Verification items for the finished model (mm, model axes). A direction names the side the tool comes from. Round coordinates to 2 decimals unless told otherwise and drop trailing zeros. Loops run counter-clockwise (first coordinate to the right, second up) from the corner with the lowest first, then second, coordinate; pieces in that order, holes last. Notation, with made-up numbers: M -11,-17.5 L -7,-17.5 A25 ccw -7,19.5 Z; hole C 43.5,-4.5 d6. An arc over 180 degrees is marked long. Answer as CSV lines item,"result".
```python
from build123d import *

# Parameters (mm, degrees)
TUBO_CUADRADO_40_X_40_X_4_1_DEPTH = 600
CROQUIS3_R                        = 4
CORTAR_EXTRUIR1_DEPTH             = 25


with BuildPart() as part:
    # Sketch1 → Tubo cuadrado 40 X 40 X 4(1) (new body)
    with BuildSketch(Plane(origin=(-300, 0, 0), x_dir=(0, 0, -1), z_dir=(1, 0, 0))):
        with BuildLine():
            Line((-12, -20), (12, -20))
            ThreePointArc((12, -20), (17.656854249, -17.656854249), (20, -12))
            Line((20, -12), (20, 12))
            ThreePointArc((20, 12), (17.656854249, 17.656854249), (12, 20))
            Line((12, 20), (-12, 20))
            ThreePointArc((-12, 20), (-17.656854249, 17.656854249), (-20, 12))
            Line((-20, 12), (-20, -12))
            ThreePointArc((-20, -12), (-17.656854249, -17.656854249), (-12, -20))
        make_face()
        with BuildLine():
            Line((-12, -16), (12, -16))
            ThreePointArc((12, -16), (14.828427125, -14.828427125), (16, -12))
            Line((16, -12), (16, 12))
            ThreePointArc((16, 12), (14.828427125, 14.828427125), (12, 16))
            Line((12, 16), (-12, 16))
            ThreePointArc((-12, 16), (-14.828427125, 14.828427125), (-16, 12))
            Line((-16, 12), (-16, -12))
            ThreePointArc((-16, -12), (-14.828427125, -14.828427125), (-12, -16))
        make_face(mode=Mode.SUBTRACT)
    extrude(amount=TUBO_CUADRADO_40_X_40_X_4_1_DEPTH)

    # Croquis3 → Cortar-Extruir1 (cut, symmetric)
    with BuildSketch(Plane.XY):
        with Locations((-270, 0)):
            Circle(CROQUIS3_R)
        with Locations((-230, 0)):
            Circle(CROQUIS3_R)
        with Locations((220, 0)):
            Circle(CROQUIS3_R)
        with Locations((245, 0)):
            Circle(CROQUIS3_R)
        with Locations((270, 0)):
            Circle(CROQUIS3_R)
    extrude(amount=CORTAR_EXTRUIR1_DEPTH, both=True, mode=Mode.SUBTRACT)


solid = part.part
```
1) Section check A-A (z = -5.5). Record the cut outline in (x, y), plus the area to 3 significant figures.
Here are the results:
outline,"M -300,-20 L 300,-20 L 300,-16 L -300,-16 Z; M -300,16 L 300,16 L 300,20 L -300,20 Z"
area,"4,800 mm^2"
2) Go/stop test with flat-tipped pins: pin 1 (6.5 mm diameter, centred on x = 270, y = 0, fed in from +Z); pin 2 (1.5 mm diameter, centred on x = 196.5, z = -14, fed in from +Y); pin 3 (1 mm diameter, centred on x = -18, y = -15, fed in from +Z). Record where each tip stops, or that it passes through.
Here are the results:
pin 1,"passes through"
pin 2,"stops at y = 19.9"
pin 3,"stops at z = 19.6"
3) Material ranges on probe 1 along Z at (x, y) = (155, -10.5); probe 2 along Y at (x, z) = (-230, 18.4), recorded low to high.
Here are the results:
probe 1,"z = -20 to -16, 16 to 20"
probe 2,"y = -16.8 to -4, 4 to 16.8"
4) Set-up check for faces 1 (the flat face through (-4, 16, 0)), 2 (the flat face through (300, 0.1, 16.4)): record each of +Z, -Z, +X, -X, +Y, -Y from which the full face is reachable in a straight line by a thin tool's end or side.
Here are the results:
face 1,"+X, -X"
face 2,"+Z, -Z, +X, +Y, -Y"
5) Section check B-B (x = -247). Record the cut outline in (y, z).
Here are the results:
outline,"M -20,-12 A8 ccw -12,-20 L 12,-20 A8 ccw 20,-12 L 20,12 A8 ccw 12,20 L -12,20 A8 ccw -20,12 Z; hole M -16,-12 A4 ccw -12,-16 L 12,-16 A4 ccw 16,-12 L 16,12 A4 ccw 12,16 L -12,16 A4 ccw -16,12 Z"
6) Draft check along Y on faces 3 (the flat face through (-4, -16, 0)), 4 (the flat face through (-4, 0, 20)), 5 (the flat face through (-4, -20, 0)), 6 (the flat face through (-4, 0, 16)). Enter one of: +Y half, -Y half, draft (parallel to the pull), parting line (faces both ways), or undercut.
Here are the results:
face 3,"undercut"
face 4,"draft"
face 5,"-Y half"
face 6,"undercut"
